Input: part model. Units: mm. Frame: model coordinates. A direction names the side the tool comes from. Coordinates: 2 decimals unless noted, no trailing zeros. Loops run counter-clockwise (first coordinate to the right, second up) from the corner with the lowest first, then second, coordinate; pieces in that order, holes last.
(1) Contact query for flat-ended pins moving along their axis: P1, Ø1, axis at x = 0.5, y = 5.5, coming from the -Z side; P2, Ø2, axis at x = -2, y = 5, coming from the -Z side; P3, Ø2, axis at y = 5, z = 2.5, coming from the -X side. Output: stop coordinate, or through.
(2) Mould query, pull axis Z, two halves, no side actions, for faces 4 (the face through (-2.312, 6.435, 0.513)), 5 (the face through (3, 12.7, 1)), 6 (the face through (4.76, 0.9, 0.62)). Classes: released by +Z, released by -Z, zero draft, split by the parting line, or undercut.
(3) Section D-D, the plane y = 1. Return loops of the section in (x, z).
(4) Section A-A, the plane z = 0. Return loops of the section in (x, y) (3 decimals).
(5) Section C-C, the plane y = 3.5. Return loops of the section in (x, z), then the cut area to 3 significant figures.
(6) Line query: L1, parallel to X at y = 9.25, z = 0; L2, parallel to Y at x = -0.75, z = 3.25; L3, parallel to Z at x = 0.5, y = 3. Output: solid intervals per line, ascending.
(7) Section B-B, the plane x = 0. Return loops of the section in (y, z) (3 decimals).
(8) Set-up query: faces 1 (the face through (-3.88, 4.83, 0.86)), 2 (the face through (-2, 8.179, -3)), 3 (the face through (-2, 0, -2)). Return all of +Z, -Z, +X, -X, +Y, -Y with unobstructed straight access to the full face (end or side cutting, diameter ignored); none if empty.
```python
from build123d import *

# Parameters (mm, degrees)
CHAMFER1_SIZE = 0.25


with BuildPart() as part:
    # Sketch2 → Revolve1 (revolve)
    with BuildSketch(Plane(origin=(0, 0, 0), x_dir=(0, 0, -1), z_dir=(1, 0, 0))):
        Polygon((2.36855, 12.7), (3.9751, 12.7), (3.9751, 8.9916), (3.175, 8.9916), (3.175, 8.1788), (3.9751, 8.1788), (3.9751, 1.5748), (4.8006, 1.5748), (4.8006, 0), (2.36855, 0), align=None)
    revolve(axis=Axis((0, -1.359924362, 0), (0, -1, 0)))

    # Chamfer1
    chamfer1_edges = [part.edges().sort_by_distance(p)[0] for p in [
        (0, 0, 4.8006),
        (0, 0, 2.36855),
        (0, 12.7, 2.36855),
        (0, 12.7, 3.9751),
    ]]
    chamfer(chamfer1_edges, length=CHAMFER1_SIZE)


solid = part.part
```
Report:
1. P1: stops at z = -3.98
1. P2: stops at z = -3.85
1. P3: stops at x = -3.68
2. face 4: undercut
2. face 5: zero draft
2. face 6: split by the parting line
3. outline: circle Ø9.6 at (0, 0); hole circle Ø4.74 at (0, 0)
4. outline: (-4.801, 0.25) - (-4.551, 0) - (-2.619, 0) - (-2.369, 0.25) - (-2.369, 12.45) - (-2.619, 12.7) - (-3.725, 12.7) - (-3.975, 12.45) - (-3.975, 8.992) - (-3.175, 8.992) - (-3.175, 8.179) - (-3.975, 8.179) - (-3.975, 1.575) - (-4.801, 1.575) - close; (2.369, 0.25) - (2.619, 0) - (4.551, 0) - (4.801, 0.25) - (4.801, 1.575) - (3.975, 1.575) - (3.975, 8.179) - (3.175, 8.179) - (3.175, 8.992) - (3.975, 8.992) - (3.975, 12.45) - (3.725, 12.7) - (2.619, 12.7) - (2.369, 12.45) - close
5. outline: circle Ø7.95 at (0, 0); hole circle Ø4.74 at (0, 0)
5. area: 32.0 mm2
6. L1: x = -3.98 to -2.37, 2.37 to 3.98
6. L2: y = 0 to 8.18, 8.99 to 12.7
6. L3: z = -3.94 to -2.32, 2.32 to 3.94
7. outline: (0, -4.551) - (0.25, -4.801) - (1.575, -4.801) - (1.575, -3.975) - (8.179, -3.975) - (8.179, -3.175) - (8.992, -3.175) - (8.992, -3.975) - (12.45, -3.975) - (12.7, -3.725) - (12.7, -2.619) - (12.45, -2.369) - (0.25, -2.369) - (0, -2.619) - close; (0, 2.619) - (0.25, 2.369) - (12.45, 2.369) - (12.7, 2.619) - (12.7, 3.725) - (12.45, 3.975) - (8.992, 3.975) - (8.992, 3.175) - (8.179, 3.175) - (8.179, 3.975) - (1.575, 3.975) - (1.575, 4.801) - (0.25, 4.801) - (0, 4.551) - close
8. face 1: +Y
8. face 2: none
8. face 3: +Z, -Z, +X, -X, -Y
